The listing builds one solid part. Answer for the finished solid, in the listing's coordinates (mm). A direction names the side the tool comes from. Round coordinates to 2 decimals unless told otherwise and drop trailing zeros. Write each loop counter-clockwise with the first axis right and the second up, starting at its lowest first coordinate (ties: lowest second). Pieces come first, ordered by that corner, then holes.
Autodesk Inventor part; units mm, degrees
ref_plane "YZ Plane" through (0, 0, 0) normal (1, 0, 0) x (0, 1, 0)
ref_plane "XZ Plane" through (0, 0, 0) normal (0, 1, 0) x (-1, 0, 0)
ref_plane "XY Plane" through (0, 0, 0) normal (0, 0, 1) x (1, 0, 0)
sketch "Esquisse1" plane through (0, 0, 0) normal (0, 1, 0) x (-1, 0, 0)
  line L0 (9.5, 2.5) -> (-9.5, 2.5)
  line L1 (-9.5, 2.5) -> (-9.5, -2.5)
  line L2 (-9.5, -2.5) -> (9.5, -2.5)
  line L3 (9.5, -2.5) -> (9.5, 2.5)
  line L4 (2.5, 9.5) -> (-2.5, 9.5)
  line L5 (-2.5, 9.5) -> (-2.5, -9.5)
  line L6 (-2.5, -9.5) -> (2.5, -9.5)
  line L7 (2.5, -9.5) -> (2.5, 9.5)
  point P0 (0, 0)
  dimension "d0" = 19
  dimension "d1" = 19
  dimension "d2" = 5
  dimension "d3" = 5
  dimension "d4" = 7
  dimension "d5" = 7
  dimension "d6" = 2.5
  dimension "d7" = 2.5
extrude "Extrusion1" add sketch "Esquisse1" along normal blind 7
sketch "Esquisse2" plane through (0, 0, 0) normal (0, -1, 0) x (1, 0, 0)
  line L0 (2.5, 9.5) -> (2.5, 2.5)
  line L1 (-2.5, 9.5) -> (2.5, 9.5)
  line L2 (-2.5, 2.5) -> (-2.5, 9.5)
  line L3 (-9.5, 2.5) -> (-2.5, 2.5)
  line L4 (-9.5, -2.5) -> (-9.5, 2.5)
  line L5 (-2.5, -2.5) -> (-9.5, -2.5)
  line L6 (-2.5, -9.5) -> (-2.5, -2.5)
  line L7 (2.5, -9.5) -> (-2.5, -9.5)
  line L8 (2.5, -2.5) -> (2.5, -9.5)
  line L9 (9.5, -2.5) -> (2.5, -2.5)
  line L10 (9.5, 2.5) -> (9.5, -2.5)
  line L11 (2.5, 2.5) -> (9.5, 2.5)
  line L12 (10.8, 3.8) -> (10.8, -3.8)
  line L13 (10.8, -3.8) -> (3.8, -3.8)
  line L14 (3.8, -3.8) -> (3.8, -10.8)
  line L15 (3.8, -10.8) -> (-3.8, -10.8)
  line L16 (-3.8, -10.8) -> (-3.8, -3.8)
  line L17 (-3.8, -3.8) -> (-10.8, -3.8)
  line L18 (-10.8, -3.8) -> (-10.8, 3.8)
  line L19 (-10.8, 3.8) -> (-3.8, 3.8)
  line L20 (-3.8, 3.8) -> (-3.8, 10.8)
  line L21 (-3.8, 10.8) -> (3.8, 10.8)
  line L22 (3.8, 10.8) -> (3.8, 3.8)
  line L23 (3.8, 3.8) -> (10.8, 3.8)
  point P0 (0, 0)
  dimension "d10" = 1.3
extrude "Extrusion2" add sketch "Esquisse2" along normal blind 1.5 contours L0 L11 L10 L9 L8 L7 L6 L5 L4 L3 L2 L1 | L12 L13 L14 L15 L16 L17 L18 L19 L20 L21 L22 L23
fillet "Congé1" radius 2 4 edges at (0, 7, 9.5) (9.5, 7, 0) (0, 7, -9.5) (-9.5, 7, 0)
fillet "Congé2" radius 0.5 24 edges at (2.5, 6.4142, 8.9142) (2.5, 2.5, 9.5) (2.5, 7, 5) (8.9142, 6.4142, 2.5) (9.5, 2.5, 2.5) (5, 7, 2.5) (8.9142, 6.4142, -2.5) (9.5, 2.5, -2.5) (5, 7, -2.5) (2.5, 6.4142, -8.9142) (2.5, 2.5, -9.5) (2.5, 7, -5) (-2.5, 6.4142, -8.9142) (-2.5, 2.5, -9.5) (-2.5, 7, -5) (-8.9142, 6.4142, -2.5) (-9.5, 2.5, -2.5) (-5, 7, -2.5) (-8.9142, 6.4142, 2.5) (-9.5, 2.5, 2.5) (-5, 7, 2.5) (-2.5, 6.4142, 8.9142) (-2.5, 2.5, 9.5) (-2.5, 7, 5)
fillet "Congé3" radius 0.5 12 edges at (10.8, -0.75, -3.8) (10.8, -0.75, 3.8) (3.8, -0.75, -3.8) (3.8, -0.75, -10.8) (-3.8, -0.75, -10.8) (-3.8, -0.75, -3.8) (-10.8, -0.75, -3.8) (-10.8, -0.75, 3.8) (-3.8, -0.75, 3.8) (-3.8, -0.75, 10.8) (3.8, -0.75, 10.8) (3.8, -0.75, 3.8)
sketch "Esquisse3" plane through (0, 7, 0) normal (0, 1, 0) x (1, 0, 0)
  line L0 (1.1, -4.5) -> (-1.2682, -4.5)
  line L1 (-1.2682, -4.5) -> (0, -6.5)
  line L2 (1.1, -4.5) -> (0, -6.5)
  line L3 (2.5, -7.5) -> (2.5, -2.5)
  line L4 (-2, -9.5) -> (2, -9.5)
  line L5 (-4.5, -1.1) -> (-4.5, 1.2682)
  line L6 (-4.5, 1.2682) -> (-6.5, 0)
  line L7 (-4.5, -1.1) -> (-6.5, 0)
  line L8 (-1.1, 4.5) -> (1.2682, 4.5)
  line L9 (1.2682, 4.5) -> (0, 6.5)
  line L10 (-1.1, 4.5) -> (0, 6.5)
  line L11 (4.5, 1.1) -> (4.5, -1.2682)
  line L12 (4.5, -1.2682) -> (6.5, 0)
  line L13 (4.5, 1.1) -> (6.5, 0)
  point P0 (0, 0)
  point P1 (0, 0)
  point P2 (0, 0)
  point P3 (0, 0)
  dimension "d18" = 1.1
  dimension "d19" = 2.5
  dimension "d20" = 3
  dimension "d21" = 5
  dimension "d24" = 360
extrude "Extrusion3" cut sketch "Esquisse3" against normal blind 0.2
equation "\"d1\" = d0"
equation "\"d3\" = d2"
equation "\"d4\" = -0.5 * d2 + 0.5 * d0"
equation "\"d5\" = d4"
properties part number "Cross" material "Plastique ABS"
1. A tool of negligible diameter and unlimited length cuts with its end or side. For faces 1 (the face through (-6, 3, 2.5)), 2 (the face through (0, 2, -9.5)), 3 (the face through (-2.5, 3, -6)), 4 (the face through (3.8, -1, -7)), from which of +Z, -Z, +X, -X, +Y, -Y can it reach the whole face along a straight path? Write none if from no direction.
Geometry says:
face 1: +Z, -X, +Y
face 2: -Z, +X, -X, +Y
face 3: -Z, -X, +Y
face 4: -Z, +X, +Y, -Y
2. Section C-C on x = -3 is taken. Determine the outline of the cut face in (y, z).
Geometry says:
outline: (-1.5, -10.8) - (0, -10.8) - (0, -2.5) - (6.5, -2.5) arc R0.5 ccw to (7, -2) - (7, 2) arc R0.5 ccw to (6.5, 2.5) - (0, 2.5) - (0, 10.8) - (-1.5, 10.8) - close
3. Straight lines are drawn through the part: line 1 along X through (y, z) = (1.25, -1.75); line 2 along X through (y, z) = (0.5, 8.75). For each, find the intervals that lie inside material, in ascending order.
Geometry says:
line 1: x = -9.5 to 9.5
line 2: x = -2.5 to 2.5
4. Section A-A on z = 7 is taken. Determine the outline of the cut face in (x, y).
Geometry says:
outline: (-3.8, -1.5) - (3.8, -1.5) - (3.8, 0) - (2.5, 0) - (2.5, 6.5) arc R0.5 ccw to (2, 7) - (-2, 7) arc R0.5 ccw to (-2.5, 6.5) - (-2.5, 0) - (-3.8, 0) - close
5. Section B-B on y = 2.25 is taken. Determine the outline of the cut face in (x, z), plus the area to 3 significant figures.
Geometry says:
outline: (-9.5, -2) arc R0.5 ccw to (-9, -2.5) - (-2.5, -2.5) - (-2.5, -9) arc R0.5 ccw to (-2, -9.5) - (2, -9.5) arc R0.5 ccw to (2.5, -9) - (2.5, -2.5) - (9, -2.5) arc R0.5 ccw to (9.5, -2) - (9.5, 2) arc R0.5 ccw to (9, 2.5) - (2.5, 2.5) - (2.5, 9) arc R0.5 ccw to (2, 9.5) - (-2, 9.5) arc R0.5 ccw to (-2.5, 9) - (-2.5, 2.5) - (-9, 2.5) arc R0.5 ccw to (-9.5, 2) - close
area: 165 mm2
6. Section D-D on z = -6 is taken. Determine the outline of the cut face in (x, y) (3 decimals), plus the area to 3 significant figures.
Geometry says:
outline: (-3.8, -1.5) - (3.8, -1.5) - (3.8, 0) - (2.5, 0) - (2.5, 6.5) arc R0.5 ccw to (2, 7) - (0.317, 7) - (0.317, 6.8) - (-0.275, 6.8) - (-0.275, 7) - (-2, 7) arc R0.5 ccw to (-2.5, 6.5) - (-2.5, 0) - (-3.8, 0) - close
area: 46.2 mm2
7. Given pin 1 (1.2 mm diameter, centred on y = 1.5, z = -1, fed in from -X); pin 2 (2 mm diameter, centred on y = 3, z = 1.5, fed in from +X); pin 3 (5 mm diameter, centred on y = 3, z = -7, fed in from +X), each flat-ended and moving along its own axis, determine where each tip first touches the part or whether it passes through.
Geometry says:
pin 1: stops at x = -9.5
pin 2: stops at x = 9.5
pin 3: stops at x = 2.5
